from build123d import *

# Parameters (mm, degrees)
EXTRUDE_1_DEPTH     = 1
SKETCH_2_R          = 2.5
SKETCH_2_R_2        = 1.75
EXTRUDE_2_DEPTH     = 4
SKETCH_3_R          = 1
CUT_EXTRUDE_1_DEPTH = 4
SKETCH_4_R          = 1.5
CUT_EXTRUDE_2_DEPTH = 0.5


with BuildPart() as part:
    # 草图1 → 凸台-拉伸1 (new body)
    with BuildSketch(Plane(origin=(0, 0, 0), x_dir=(1, 0, 0), z_dir=(0, 1, 0))):
        with BuildLine():
            Line((-15, 2.5), (15, 2.5))
            ThreePointArc((15, 2.5), (17.5, 0), (15, -2.5))
            Line((15, -2.5), (-15, -2.5))
            ThreePointArc((-15, -2.5), (-17.5, 0), (-15, 2.5))
        make_face()
    extrude(amount=EXTRUDE_1_DEPTH)

    # 草图2 → 凸台-拉伸2 (add)
    with BuildSketch(Plane(origin=(0, 0, 0), x_dir=(1, 0, 0), z_dir=(0, 1, 0))):
        with Locations(Location((0, 0, 0), (0, 0, 270))):
            Circle(SKETCH_2_R)
        with Locations(Location((0, 0, 0), (0, 0, 270))):
            Circle(SKETCH_2_R_2, mode=Mode.SUBTRACT)
    extrude(amount=EXTRUDE_2_DEPTH)

    # 草图3 → 切除-拉伸1 (cut)
    with BuildSketch(Plane(origin=(0, 0, 0), x_dir=(1, 0, 0), z_dir=(0, 1, 0))):
        with Locations(Location((0, 0, 0), (0, 0, 270))):
            Circle(SKETCH_3_R)
    extrude(amount=CUT_EXTRUDE_1_DEPTH, mode=Mode.SUBTRACT)

    # 草图4 → 切除-拉伸2 (cut)
    with BuildSketch(Plane(origin=(0, 0, 0), x_dir=(1, 0, 0), z_dir=(0, 1, 0))):
        with Locations(Location((0, 0, 0), (0, 0, 270))):
            Circle(SKETCH_4_R)
    extrude(amount=CUT_EXTRUDE_2_DEPTH, mode=Mode.SUBTRACT)


solid = part.part
Model file for the job. Use its own axes, mm. A direction names the side the tool comes from. Give positions to 0.01 mm unless a question says otherwise; leave off trailing zeros. Order: outer loops, then holes, each group sorted by start corner. A loop starts at its lowest first (then second) coordinate and runs counter-clockwise, first axis right, second up. Notation, with made-up numbers: (-11.5, 34.5) -> (39.5, 34.5) arc R13 ccw to (39.5, 46.5) -> close; hole circle Ø5 at (33, 42). An arc over 180 degrees is marked (long way). Use CSV: the item, a comma, the result in double quotes.
1. Drop a flat-ended pin along its axis: pin 1 (2.5 mm diameter, centred on x = 0, z = 0, fed in from +Y). Give the stop position or say it passes through.
Outcome:
pin 1,"y = 1"
2. Band-saw the part on B-B, the plane y = 2.95. Give the cut face in (x, z).
Outcome:
outline,"circle Ø5 at (0, 0); hole circle Ø3.5 at (0, 0)"
3. Mould opens along X. For faces 3 (the cylindrical face through (-2.44, 2.48, -0.54)), 4 (the flat face through (2, 4, 1)), 5 (the flat face through (-1, 1, 1)), 6 (the cylindrical face through (0.45, 0.25, 1.43)) say: +X half, -X half, draft (parallel to the pull), parting line (faces both ways), or undercut.
Outcome:
face 3,"parting line"
face 4,"draft"
face 5,"undercut"
face 6,"undercut"
4. Drill centre lines: line 1 along Z through (x, y) = (0, 0.7); line 2 along Z through (x, y) = (0, 1.1); line 3 along X through (y, z) = (0.2, 0). Where is each one in solid material? Low to high. Write a range as from..to.
Outcome:
line 1,"-2.5..-1, 1..2.5"
line 2,"-2.5..-1.75, 1.75..2.5"
line 3,"-17.5..-1.5, 1.5..17.5"
5. Band-saw the part on A-A, the plane z = 0. Give the cut face in (x, y), then the cut area to 3 significant figures.
Outcome:
outline,"(-17.5, 0) -> (-1.5, 0) -> (-1.5, 0.5) -> (-1, 0.5) -> (-1, 1) -> (-1.75, 1) -> (-1.75, 4) -> (-2.5, 4) -> (-2.5, 1) -> (-17.5, 1) -> close; (1, 0.5) -> (1.5, 0.5) -> (1.5, 0) -> (17.5, 0) -> (17.5, 1) -> (2.5, 1) -> (2.5, 4) -> (1.75, 4) -> (1.75, 1) -> (1, 1) -> close"
area,"37.0 mm²"
6. 3-axis set-ups, long thin cutter, end or side, ignore diameter. For faces 1 (the cylindrical face through (-0.976, 0.746, -0.217)), 2 (the cylindrical face through (-1.71, 2.48, -0.38)): which of +Z, -Z, +X, -X, +Y, -Y reach the whole face in a straight line?
Outcome:
face 1,"+Y, -Y"
face 2,"+Y"
7. Band-saw the part on C-C, the plane x = 5. Give the cut face in (y, z), then the cut area to 3 significant figures.
Outcome:
outline,"(0, -2.5) -> (1, -2.5) -> (1, 2.5) -> (0, 2.5) -> close"
area,"5.00 mm²"
